```python
from build123d import *

# Parameters (mm, degrees)
F0_W     = 35
F0_H     = 8
F0_R     = 1.75
F0_R_2   = 1.875
F0_R_3   = 2
F0_R_4   = 2.125
F0_R_5   = 2.25
F1_DEPTH = 2
F2_DEPTH = 2
F3_DEPTH = 5
F4_R     = 3


with BuildPart() as f1:
    # F0 (on Front) → F1 (new body)
    with BuildSketch(Plane.XZ):
        with Locations((17.5, -4)):
            Rectangle(F0_W, F0_H)
        with Locations((4.12062, -3.782185)):
            Circle(F0_R, mode=Mode.SUBTRACT)
        with Locations((10.021019, -3.722706)):
            Circle(F0_R_2, mode=Mode.SUBTRACT)
        with Locations((16.803088, -3.65434)):
            Circle(F0_R_3, mode=Mode.SUBTRACT)
        with Locations((24.195543, -3.784031)):
            Circle(F0_R_4, mode=Mode.SUBTRACT)
        with Locations((31.113254, -3.646227)):
            Circle(F0_R_5, mode=Mode.SUBTRACT)
    extrude(amount=F1_DEPTH)

    # F0 (on Front) → F2 (join)
    with BuildSketch(Plane.XZ):
        with Locations((17.5, -12)):
            Rectangle(F0_W, F0_H)
        with Locations((4.12062, -12.217815)):
            Circle(F0_R, mode=Mode.SUBTRACT)
        with Locations((10.021019, -12.277294)):
            Circle(F0_R_2, mode=Mode.SUBTRACT)
        with Locations((16.803088, -12.34566)):
            Circle(F0_R_3, mode=Mode.SUBTRACT)
        with Locations((24.195543, -12.215969)):
            Circle(F0_R_4, mode=Mode.SUBTRACT)
        with Locations((31.113254, -12.353773)):
            Circle(F0_R_5, mode=Mode.SUBTRACT)
    extrude(amount=F2_DEPTH)

    # F0 (on Front) → F3 (join)
    with BuildSketch(Plane.XZ):
        with Locations((31.113254, -12.353773)):
            Circle(F0_R_5)
        with Locations((24.195543, -12.215969)):
            Circle(F0_R_4)
        with Locations((16.803088, -12.34566)):
            Circle(F0_R_3)
        with Locations((10.021019, -12.277294)):
            Circle(F0_R_2)
        with Locations((4.12062, -12.217815)):
            Circle(F0_R)
    extrude(amount=F3_DEPTH)

    # F4
    f4_edges = [f1.edges().sort_by_distance(p)[0] for p in [
        (0, -1, 0),
        (0, -1, -16),
        (35, -1, -16),
        (35, -1, 0),
    ]]
    fillet(f4_edges, radius=F4_R)


solid = f1.part
```
Could you check a few things on this model? Use its own coordinates, in mm. A direction names the side the tool comes from. Coordinates: 2 decimals unless noted, no trailing zeros. Write each loop counter-clockwise with the first axis right and the second up, starting at its lowest first coordinate (ties: lowest second). Pieces come first, ordered by that corner, then holes. Notation, with made-up numbers: M 26,-20 L 44,-20 A17 cw 44,12 Z; hole C 82,0 d3. An arc over 180 degrees is marked long. Answer as CSV lines item,"result". Start each with the question number.
1) I want a section at C-C, the plane y = -1.15. Please give me the cut outline in (x, z) (3 decimals), and give its area (3 significant figures).
2) For faces 1 (the cylindrical face through (0.86, -1.01, -0.9)), 2 (the cylindrical face through (17.88, -3.48, -10.66)), which set-ups out of +Z, -Z, +X, -X, +Y, -Y let a thin tool reach every point of the face, with its end or its side?
3) For P1, Ø3, axis at x = 6.5, y = -4, coming from the +Z side; P2, Ø3, axis at x = 8.5, z = -6, coming from the -Y side, each with a flat end and sliding along its axis, tell me the tip position at first contact or that it passes through.
4) We'd pull the mould along X, two halves only. Please class faces 3 (the flat face through (35, -1, -8)), 4 (the flat face through (4, -5, -12)), 5 (the cylindrical face through (17.88, -0.99, -1.97)): +X half, -X half, draft (parallel to the pull), parting line (faces both ways), or undercut.
5) I want a section at B-B, the plane z = -5. Please give me the cut outline in (x, y), and give its area (3 significant figures).
6) Please list where these lines run through material, in increasing order: line 1 (X direction, y = -0.6, z = -2.25); line 2 (Y direction, x = 22, z = -5); line 3 (X direction, y = -0.4, z = -3.5). Write a range as from..to.
7) I want a section at D-D, the plane y = -4.65. Please give me the cut outline in (x, z) (3 decimals).
8) I want a section at A-A, the plane x = 23.5. Please give me the cut outline in (y, z).
Data:
1,outline,"M 0,-13 A3 ccw 3,-16 L 32,-16 A3 ccw 35,-13 L 35,-3 A3 ccw 32,0 L 3,0 A3 ccw 0,-3 Z; hole C 4.121,-3.782 d3.5; hole C 10.021,-3.723 d3.75; hole C 16.803,-3.654 d4; hole C 24.196,-3.784 d4.25; hole C 31.113,-3.646 d4.5"
1,area,"489 mm^2"
2,face 1,"+Z, -X, +Y, -Y"
2,face 2,"-Y"
3,P1,"stops at z = -10.7"
3,P2,"stops at y = -2"
4,face 3,"+X half"
4,face 4,"draft"
4,face 5,"undercut"
5,outline,"M 0,-2 L 2.86,-2 L 2.86,0 L 0,0 Z; M 5.38,-2 L 8.65,-2 L 8.65,0 L 5.38,0 Z; M 11.39,-2 L 15.32,-2 L 15.32,0 L 11.39,0 Z; M 18.28,-2 L 22.45,-2 L 22.45,0 L 18.28,0 Z; M 25.94,-2 L 29.32,-2 L 29.32,0 L 25.94,0 Z; M 32.91,-2 L 35,-2 L 35,0 L 32.91,0 Z"
5,area,"39.4 mm^2"
6,line 1,"x = 0.1..3.28, 4.97..8.86, 11.18..15.38, 18.23..22.73, 25.67..29.35, 32.88..34.9"
6,line 2,"y = -2..0"
6,line 3,"x = 0..2.39, 5.85..8.16, 11.88..14.81, 18.8..22.09, 26.3..28.87, 33.36..35"
7,outline,"C 4.121,-12.218 d3.5; C 10.021,-12.277 d3.75; C 16.803,-12.346 d4; C 24.196,-12.216 d4.25; C 31.113,-12.354 d4.5"
8,outline,"M -5,-14.22 L -2,-14.22 L -2,-16 L 0,-16 L 0,-5.79 L -2,-5.79 L -2,-10.21 L -5,-10.21 Z; M -2,-1.78 L 0,-1.78 L 0,0 L -2,0 Z"
